CAD build for the part. Positions are in the model's coordinates, mm. A direction names the side the tool comes from. Give positions to 0.01 mm unless a question says otherwise; leave off trailing zeros. Write each loop counter-clockwise with the first axis right and the second up, starting at its lowest first coordinate (ties: lowest second). Pieces come first, ordered by that corner, then holes. Notation, with made-up numbers: (64, -20) -> (118, -20) arc R26 cw to (118, 1) -> close; hole circle Ø3 at (80.5, 13). An arc over 180 degrees is marked (long way). Answer in a Markdown table with one row per item. Add a question column.
Autodesk Inventor part; units mm, degrees
ref_plane "РабПлоскость1" through (-69.5, 86.25, 34) normal (0, 0, -1) x (0, -1, 0)
ref_plane "YZ Plane" through (0, 0, 0) normal (1, 0, 0) x (0, 1, 0)
ref_plane "XZ Plane" through (0, 0, 0) normal (0, 1, 0) x (-1, 0, 0)
sketch "Эскиз1" plane through (0, 0, 0) normal (0, 0, 1) x (1, 0, 0)
  line L0 (40, -86.25) -> (-40, -86.25)
  line L1 (-40, -86.25) -> (-40, 86.25)
  line L2 (-40, 86.25) -> (40, 86.25)
  line L3 (40, 86.25) -> (40, -86.25)
  line L4 (40, -86.25) -> (-40, 86.25) construction
  line L5 (-40, -86.25) -> (40, 86.25) construction
  point P0 (0, 0)
  dimension "d0" = 80
  dimension "d1" = 172.5
extrude "Выдавливание1" add sketch "Эскиз1" along normal blind 3
sketch "Эскиз2" plane through (-40, -86.25, 0) normal (-1, 0, 0) x (0, 0, 1)
  line L0 (0, 172.5) -> (39, 172.5)
  line L1 (39, 172.5) -> (39, 0)
  line L2 (39, 0) -> (0, 0)
  line L3 (0, 0) -> (0, 172.5)
  dimension "d4" = 39
extrude "Выдавливание2" add sketch "Эскиз2" along normal blind 3
sketch "Эскиз3" plane through (-43, -86.25, 0) normal (-1, 0, 0) x (0, 0, 1)
  line L0 (3, 0) -> (39, 0)
  line L1 (39, 172.5) -> (3, 172.5)
  line L2 (39, 0) -> (34, 0)
  line L3 (34, 0) -> (34, 172.5)
  line L4 (34, 172.5) -> (39, 172.5)
  line L5 (39, 172.5) -> (39, 0)
  point P0 (0, 86.25)
  point P1 (34, 0)
  dimension "d7" = 5
extrude "Выдавливание3" add sketch "Эскиз3" along normal blind 26.5
sketch "Эскиз4" plane through (-43, -86.25, 34) normal (0, 0, -1) x (-1, 0, 0)
  point P0 (-43, 86.25)
sketch "Эскиз5" plane through (-43, -86.25, 34) normal (0, 0, -1) x (-1, 0, 0)
  circle A0 centre (13, 30.25) radius 1.85
  circle A1 centre (13, 142.25) radius 1.85
  point P0 (-43, 86.25)
extrude "Выдавливание4" cut sketch "Эскиз5" against normal blind 26.5
sketch "Эскиз6" plane through (40, 86.25, 3) normal (0, 1, 0) x (1, 0, 0)
  line L0 (0, 3) -> (-83, 3)
  line L1 (-83, -31) -> (-109.5, -31)
  line L2 (-83, 3) -> (-109.5, -31)
  line L3 (-83, 3) -> (-83, -31)
  line L4 (-83, 3) -> (-83, -31)
  line L5 (-80, 0) -> (-80, -36)
  point P0 (-40, 3)
extrude "Выдавливание5" add sketch "Эскиз6" against normal up to surface (172.5 mm away)
ref_plane "РабПлоскость1" through (-69.5, 86.25, 34) normal (0, 0, -1) x (0, -1, 0)
sketch "Эскиз7" plane through (-69.5, 86.25, 34) normal (0, 0, -1) x (0, -1, 0)
  circle A0 centre (142.25, -13.5) radius 1.85
  circle A1 centre (30.25, -13.5) radius 1.85
  circle A2 centre (30.25, -13.5) radius 1.85
  circle A3 centre (30.25, -13.5) radius 5
  circle A4 centre (142.25, -13.5) radius 1.85
  circle A5 centre (142.25, -13.5) radius 5
  point P0 (86.25, -69.5)
  dimension "d15" = 10
  dimension "d16" = 10
extrude "Выдавливание6" cut sketch "Эскиз7" along normal blind 36.75 contours A0 | A1 | A3 | A5
fillet "Сопряжение1" radius 10 2 edges at (-40, 0, 3) (-43, 0, 0)
fillet "Сопряжение2" radius 10 1 edges at (-69.5, 0, 34)
sketch "Эскиз8" plane through (0, 0, 0) normal (0, 0, -1) x (-1, 0, 0)
  line L0 (-35, 76.25) -> (40, 76.25)
  line L1 (-35, -76.25) -> (-35, 76.25)
  line L2 (40, -76.25) -> (-35, -76.25)
  line L3 (-40, -86.25) -> (38.1155, -86.25)
  line L4 (-40, -86.25) -> (-40, 86.25)
  line L5 (-40, 86.25) -> (38.1155, 86.25)
  circle A0 centre (-30, 81.25) radius 2
  circle A1 centre (-30, -81.25) radius 2
  point P0 (0, 0)
  dimension "d21" = 4
  dimension "d22" = 5
  dimension "d23" = 10
  dimension "d24" = 10
  dimension "d25" = 4
  dimension "d26" = 5
  dimension "d27" = 10
extrude "Выдавливание7" cut sketch "Эскиз8" against normal blind 10
equation "\"d16\" = d15"
properties part number "000.003.002 - Крышка"
Item 1: Slice it at C-C, the plane y = -4. List the corners of the cut face in (x, z), then the cut area to 3 significant figures.
Item 2: Slice it at D-D, the plane z = 29.5. List the corners of the cut face in (x, y).
Item 3: Slice it at B-B, the plane y = -81.25. List the corners of the cut face in (x, z).
Item 4: Mould opens along Y. For faces 4 (the face through (-43, 86.25, 20)), 5 (the face through (-43, -86.25, 18)), 6 (the face through (-51.043, 56.651, 24.927)), 7 (the face through (-68.94, 1.21, 34.14)) say: released by +Y, released by -Y, zero draft, split by the parting line, or undercut.
Item 5: Probe L1, parallel to Y at x = -56, z = 35; L2, parallel to Y at x = -52.5, z = 19; L3, parallel to Z at x = -16.5, y = 54. List the from-to ranges inside material, lowest first. Write a range as from..to.
Item 6: Drop flat-ended pins along their axis: pin 1 Ø4 at (y, z) = (23, 4) entering from -X; pin 2 Ø13 at (y, z) = (18.5, 28.5) entering from +X; pin 3 Ø2 at (y, z) = (-53.5, 8) entering from +X; pin 4 Ø3 at (x, y) = (-56, 56) entering from +Z. Give the stop position or say it passes through.
Item 7: Slice it at A-A, the plane x = 30. List the corners of the cut face in (y, z).
Item 8: Which spindle directions (+Z, -Z, +X, -X, +Y, -Y) get a long thin tool onto all of the face, cutting with end or side? Do faces 1 (the face through (5, 1, 3)), 2 (the face through (-56.1, -58.2, 34)), 3 (the face through (28.925, 82.936, 1.479)). Say none if no direction does.
Answer key:
| question | item | result |
|---|---|---|
| 1 | outline | (-69.5, 37.44) arc R10 ccw to (-67.39, 31.29) -> (-46, 3.85) arc R10 ccw to (-38.12, 0) -> (40, 0) -> (40, 3) -> (-30, 3) arc R10 cw to (-40, 13) -> (-40, 39) -> (-69.5, 39) -> close |
| 1 | area | 957 mm² |
| 2 | outline | (-65.99, -86.25) -> (-40, -86.25) -> (-40, 86.25) -> (-65.99, 86.25) -> close; hole circle Ø10 at (-56, -56); hole circle Ø10 at (-56, 56) |
| 3 | outline | (-69.5, 37.44) arc R10 ccw to (-67.39, 31.29) -> (-46, 3.85) arc R10 ccw to (-38.12, 0) -> (28, 0) -> (28, 3) -> (-30, 3) arc R10 cw to (-40, 13) -> (-40, 39) -> (-69.5, 39) -> close; (32, 0) -> (40, 0) -> (40, 3) -> (32, 3) -> close |
| 4 | face 4 | released by +Y |
| 4 | face 5 | released by -Y |
| 4 | face 6 | undercut |
| 4 | face 7 | zero draft |
| 5 | L1 | y = -86.25..-57.85, -54.15..54.15, 57.85..86.25 |
| 5 | L2 | y = -86.25..-59.57, -52.43..52.43, 59.57..86.25 |
| 5 | L3 | z = 0..3 |
| 6 | pin 1 | stops at x = -47.68 |
| 6 | pin 2 | stops at x = -40 |
| 6 | pin 3 | stops at x = -38 |
| 6 | pin 4 | passes through |
| 7 | outline | (-86.25, 0) -> (-83.25, 0) -> (-83.25, 3) -> (-86.25, 3) -> close; (-79.25, 0) -> (79.25, 0) -> (79.25, 3) -> (-79.25, 3) -> close; (83.25, 0) -> (86.25, 0) -> (86.25, 3) -> (83.25, 3) -> close |
| 8 | face 1 | +Z, +X, +Y, -Y |
| 8 | face 2 | -Z |
| 8 | face 3 | +Z, -Z |
